Model file for the job. Use its own axes, mm. A direction names the side the tool comes from. Coordinates: 2 decimals unless noted, no trailing zeros. Loops run counter-clockwise (first coordinate to the right, second up) from the corner with the lowest first, then second, coordinate; pieces in that order, holes last. Notation, with made-up numbers: M 10.25,47.5 L 17.25,47.5 A8 cw 17.25,56.5 Z; hole C 32.25,-32 d1. An arc over 180 degrees is marked long. One line per question, with ' | ' between items. Start each with the question number.
```python
from build123d import *

# Parameters (mm, degrees)
SKETCH_1_R          = 30
EXTRUDE_1_DEPTH     = 10
CUT_EXTRUDE_1_DEPTH = 10
FILLET_1_R          = 2
FILLET_2_R          = 5
SKETCH_3_R          = 1.65
CUT_EXTRUDE_2_DEPTH = 10
SKETCH_4_R          = 30
SKETCH_4_R_2        = 29.75
EXTRUDE_2_DEPTH     = 10


with BuildPart() as part:
    # 草图1 → 凸台-拉伸1 (new body)
    with BuildSketch(Plane(origin=(0, 0, 0), x_dir=(1, 0, 0), z_dir=(0, 1, 0))):
        with Locations(Location((0, 0, 0), (0, 0, 270))):
            Circle(SKETCH_1_R)
    extrude(amount=EXTRUDE_1_DEPTH)

    # 草图2 → 切除-拉伸1 (cut)
    with BuildSketch(Plane.XZ):
        with BuildLine():
            Line((10.93428015, 1), (30.93428015, 1))
            Line((30.93428015, 1), (30.93428015, -1))
            Line((30.93428015, -1), (10.93428015, -1))
            ThreePointArc((10.93428015, -1), (4.9, 0), (10.93428015, 1))
        make_face()
    extrude(amount=-CUT_EXTRUDE_1_DEPTH, mode=Mode.SUBTRACT)

    # 圆角1
    fillet_1_edges = [part.edges().sort_by_distance(p)[0] for p in [
        (10.93428015, 5, 1),
        (10.93428015, 5, -1),
    ]]
    fillet(fillet_1_edges, radius=FILLET_1_R)

    # 圆角2
    fillet_2_edges = [part.edges().sort_by_distance(p)[0] for p in [
        (29.983328701, 5, 1),
        (29.983328701, 5, -1),
    ]]
    fillet(fillet_2_edges, radius=FILLET_2_R)

    # 草图3 → 切除-拉伸2 (cut)
    with BuildSketch(Plane.XZ):
        with Locations(Location((-5, 0, 0), (0, 0, 270))):
            Circle(SKETCH_3_R)
        with Locations(Location((2.5, 4.330127019, 0), (0, 0, 270))):
            Circle(SKETCH_3_R)
        with Locations(Location((2.5, -4.330127019, 0), (0, 0, 270))):
            Circle(SKETCH_3_R)
    extrude(amount=-CUT_EXTRUDE_2_DEPTH, mode=Mode.SUBTRACT)

    # 草图4 → 凸台-拉伸2 (add)
    with BuildSketch(Plane.XZ):
        with Locations(Location((0, 0, 0), (0, 0, 90))):
            Circle(SKETCH_4_R)
        Circle(SKETCH_4_R_2, mode=Mode.SUBTRACT)
    extrude(amount=-EXTRUDE_2_DEPTH)


solid = part.part
```
(1) Drill centre lines: line 1 (X direction, y = 6, z = 0); line 2 (Z direction, x = 8, y = 7.75); line 3 (Z direction, x = 26.5, y = 6). Where is each one in solid material? Low to high. Write a range as [from, to].
(2) Band-saw the part on B-B on x = 7.5. Write the cut outline in (y, z), then the cut area to 3 significant figures.
(3) Band-saw the part on D-D on x = -5. Write the cut outline in (y, z), then the cut area to 3 significant figures.
(4) 3-axis set-ups, long thin cutter, end or side, ignore diameter. For faces 4 (the face through (18, 5, 1)), 5 (the face through (0, 10, 0)): which of +Z, -Z, +X, -X, +Y, -Y reach the whole face in a straight line?
(5) Two-plate mould, pull along X, no slides. Class faces 1 (the face through (0, 0, 0)), 2 (the face through (4.9, 4.9, -0.1)), 3 (the face through (-16.6, 4.93, -24.99)): pulls with the +X half, pulls with the -X half, needs draft (parallel to the pull), parting line crosses it, or undercut.
(6) Band-saw the part on C-C on y = 0.75. Write the cut outline in (x, z).
(7) Pin check, flat tips, straight feed: P1, Ø2, axis at x = -24, z = -22, coming from the -Y side; P2, Ø3, axis at x = 18, y = 3.5, coming from the -Z side; P3, Ø5, axis at x = 16, y = 4, coming from the +Z side; P4, Ø5, axis at y = 5, z = -6.5, coming from the -X side. Stop position of each tip, or through.
(8) Band-saw the part on A-A on z = 0. Write the cut outline in (x, y), then the cut area to 4 significant figures.
Computed values:
1) line 1: [-30, -6.65], [-3.35, 4.9], [29.75, 30] | line 2: [-28.91, -3.1], [3.1, 28.91] | line 3: [-14.06, -1.53], [1.53, 14.06]
2) outline: M 0,-29.05 L 10,-29.05 L 10,-3.06 L 0,-3.06 Z; M 0,3.06 L 10,3.06 L 10,29.05 L 0,29.05 Z | area: 520 mm^2
3) outline: M 0,-29.58 L 10,-29.58 L 10,-1.65 L 0,-1.65 Z; M 0,1.65 L 10,1.65 L 10,29.58 L 0,29.58 Z | area: 559 mm^2
4) face 4: +Y, -Y | face 5: +Z, -Z, +X, -X, +Y
5) face 1: needs draft | face 2: undercut | face 3: parting line crosses it
6) outline: C 0,0 d60; hole C -5,0 d3.3; hole C 2.5,-4.33 d3.3; hole C 2.5,4.33 d3.3; hole M 10.51,-1.82 A2 cw 12.12,-1 L 24.27,-1 A5 cw 29.24,-5.48 A29.75 ccw 29.24,5.48 A5 cw 24.27,1 L 12.12,1 A2 cw 10.51,1.82 A3.1 ccw long Z
7) P1: through | P2: z = -25.05 | P3: z = 26.79 | P4: x = -29.73
8) outline: M -30,0 L -6.65,0 L -6.65,10 L -30,10 Z; M -3.35,0 L 4.9,0 L 4.9,10 L -3.35,10 Z; M 29.75,0 L 30,0 L 30,10 L 29.75,10 Z | area: 318.5 mm^2
